```python
from build123d import *

# Parameters (mm, degrees)
F0_W     = 27
F0_H     = 27
F0_R     = 1.5
F1_DEPTH = 2
F2_SIZE  = 3


with BuildPart() as f1:
    # F0 (on Top) → F1 (new body)
    with BuildSketch(Plane.XY):
        Rectangle(F0_W, F0_H)
        with Locations((-10, -10)):
            Circle(F0_R, mode=Mode.SUBTRACT)
        with Locations((10, -10)):
            Circle(F0_R, mode=Mode.SUBTRACT)
        with Locations((-10, 10)):
            Circle(F0_R, mode=Mode.SUBTRACT)
        with Locations((10, 10)):
            Circle(F0_R, mode=Mode.SUBTRACT)
    extrude(amount=F1_DEPTH)

    # F2
    f2_edges = [f1.edges().sort_by_distance(p)[0] for p in [
        (13.5, -13.5, 1),
        (-13.5, -13.5, 1),
        (13.5, 13.5, 1),
        (-13.5, 13.5, 1),
    ]]
    chamfer(f2_edges, length=F2_SIZE)


solid = f1.part
```
Part model, mm, in its own coordinate system. Give positions to 0.01 mm unless a question says otherwise; leave off trailing zeros. Order: outer loops, then holes, each group sorted by start corner. A loop starts at its lowest first (then second) coordinate and runs counter-clockwise, first axis right, second up. Notation, with made-up numbers: M -24.5,-34.5 L -14.5,-34.5 A18 cw -14.5,-0.5 Z; hole C -9.75,76.25 d11. An arc over 180 degrees is marked long. Use a Markdown table: item, result. Add a question column.
(1) Saw through at A-A, the plane y = -10. Give the cut face in (x, z), and give its area (3 significant figures).
(2) Mould opens along X. For faces 1 (the face through (8.8, 9.1, 1)), 2 (the face through (-13.5, 0, 1)), 3 (the face through (0, 13.5, 1)) say: +X half, -X half, draft (parallel to the pull), parting line (faces both ways), or undercut.
(3) Drop flat-ended pins along their axis: P1, Ø5, axis at x = 10, y = 10, coming from the -Z side; P2, Ø2.5, axis at x = 10, y = -10, coming from the +Z side. Give the stop position or say it passes through.
(4) Saw through at C-C, the plane z = 0.7. Give the cut face in (x, y).
(5) Probe line 1 along Y through (x, z) = (10, 1.1); line 2 along Y through (x, z) = (8.75, 1); line 3 along Y through (x, z) = (12, 1.95). List the from-to ranges inside material, lowest first. Write a range as [from, to].
Answer key:
| question | item | result |
|---|---|---|
| 1 | outline | M -13.5,0 L -11.5,0 L -11.5,2 L -13.5,2 Z; M -8.5,0 L 8.5,0 L 8.5,2 L -8.5,2 Z; M 11.5,0 L 13.5,0 L 13.5,2 L 11.5,2 Z |
| 1 | area | 42.0 mm^2 |
| 2 | face 1 | undercut |
| 2 | face 2 | -X half |
| 2 | face 3 | draft |
| 3 | P1 | z = 0 |
| 3 | P2 | through |
| 4 | outline | M -13.5,-10.5 L -10.5,-13.5 L 10.5,-13.5 L 13.5,-10.5 L 13.5,10.5 L 10.5,13.5 L -10.5,13.5 L -13.5,10.5 Z; hole C -10,-10 d3; hole C -10,10 d3; hole C 10,-10 d3; hole C 10,10 d3 |
| 5 | line 1 | [-13.5, -11.5], [-8.5, 8.5], [11.5, 13.5] |
| 5 | line 2 | [-13.5, -10.83], [-9.17, 9.17], [10.83, 13.5] |
| 5 | line 3 | [-12, 12] |
